Here's how the part is built. I have some questions about the finished solid (model axes, mm). Give positions to 0.01 mm unless a question says otherwise; leave off trailing zeros. Write each loop counter-clockwise with the first axis right and the second up, starting at its lowest first coordinate (ties: lowest second). Pieces come first, ordered by that corner, then holes. Notation, with made-up numbers: M 87.5,4 L 96.5,4 A20 ccw 96.5,26 Z; hole C -22.5,-10 d7. An arc over 180 degrees is marked long. Use one line per item in the form item = value. Start each with the question number.
Autodesk Inventor part; units mm, degrees
ref_plane "YZ Plane" through (0, 0, 0) normal (1, 0, 0) x (0, 1, 0)
ref_plane "XZ Plane" through (0, 0, 0) normal (0, 1, 0) x (-1, 0, 0)
ref_plane "XY Plane" through (0, 0, 0) normal (0, 0, 1) x (1, 0, 0)
sketch "Sketch1" plane through (0, 0, 0) normal (0, 1, 0) x (-1, 0, 0)
  circle A0 centre (179.7843, -49) radius 2.65
  circle A1 centre (41.7843, 49) radius 2.65
  circle A2 centre (179.7843, 49) radius 2.65
  circle A3 centre (41.7843, -49) radius 2.65
  arc A4 (185.7843, 50) -> (180.7843, 55) centre (180.7843, 50) ccw
  line L0 (40.7843, 55) -> (180.7843, 55)
  arc A5 (40.7843, 55) -> (35.7843, 50) centre (40.7843, 50) ccw
  line L1 (35.7843, 12.5) -> (35.7843, 50)
  line L2 (35.7843, -50) -> (35.7843, -12.5)
  arc A6 (35.7843, -50) -> (40.7843, -55) centre (40.7843, -50) ccw
  line L3 (40.7843, -55) -> (180.7843, -55)
  arc A7 (180.7843, -55) -> (185.7843, -50) centre (180.7843, -50) ccw
  line L4 (185.7843, 50) -> (185.7843, -50)
  line L5 (35.7843, -12.5) -> (35.7843, 12.5)
  point P0 (0, 0)
  point P1 (35.7843, 55)
extrude "Extrusion1" add sketch "Sketch1" along normal blind 6
sketch "Sketch2" plane through (0, 6, 0) normal (0, 1, 0) x (1, 0, 0)
  circle A0 centre (-179.7843, 49) radius 2.65
  circle A1 centre (-179.7843, 49) radius 1.65
  circle A2 centre (-41.7843, 49) radius 2.65
  circle A3 centre (-41.7843, 49) radius 1.65
  circle A4 centre (-41.7843, -49) radius 2.65
  circle A5 centre (-41.7843, -49) radius 1.65
  circle A6 centre (-179.7843, -49) radius 2.65
  circle A7 centre (-179.7843, -49) radius 1.65
  point P0 (0, 0)
  dimension "d2" = 3.3
  dimension "d3" = 3.3
  dimension "d4" = 3.3
  dimension "d5" = 3.3
extrude "Extrusion2" add sketch "Sketch2" against normal blind 6
sketch "Sketch3" plane through (0, 0, 0) normal (0, -1, 0) x (1, 0, 0)
  circle A0 centre (-155.7843, 0) radius 9.4
  line L0 (-185.7843, 50) -> (-185.7843, -50)
  line L1 (-40.7843, 55) -> (-180.7843, 55)
  point P0 (0, 0)
  dimension "d8" = 18.8
  dimension "d9" = 30
  dimension "d10" = 55
extrude "Extrusion3" cut sketch "Sketch3" against normal blind 6
properties part number "MainHousing_BottomPlate"
1) Suppose I cut it at B-B, the plane y = 1.05. List the corners of the cut face in (x, z) for me.
2) Suppose I cut it at A-A, the plane z = 0. List the corners of the cut face in (x, y) for me.
3) Will this pin go through, and if not, where does the flat tip stop? P1, Ø2, axis at x = -41.78, z = 49, coming from the -Y side.
4) Thinking about a two-plate mould opening in X: for faces 1 (the face through (-110, 6, 1)), 2 (the face through (-181.433, 3.042, -49.073)), 3 (the face through (-185.784, 3, 1)), which applies, released by +X, released by -X, zero draft, split by the parting line, or undercut?
5) Please list where these lines run through material, in increasing order: line 1 (X direction, y = 3.05, z = 49); line 2 (Z direction, x = -156.5, y = 0.35); line 3 (X direction, y = 0.55, z = -1.5).
Checks:
q1.outline = M -185.78,-50 A5 ccw -180.78,-55 L -40.78,-55 A5 ccw -35.78,-50 L -35.78,50 A5 ccw -40.78,55 L -180.78,55 A5 ccw -185.78,50 Z; hole C -179.78,-49 d3.3; hole C -179.78,49 d3.3; hole C -155.78,0 d18.8; hole C -41.78,-49 d3.3; hole C -41.78,49 d3.3
q2.outline = M -185.78,0 L -165.18,0 L -165.18,6 L -185.78,6 Z; M -146.38,0 L -35.78,0 L -35.78,6 L -146.38,6 Z
q3.P1 = through
q4.face_1 = zero draft
q4.face_2 = undercut
q4.face_3 = released by -X
q5.line_1 = -185.78 to -181.43, -178.13 to -43.43, -40.13 to -35.78
q5.line_2 = -55 to -9.37, 9.37 to 55
q5.line_3 = -185.78 to -165.06, -146.5 to -35.78
